Could you check a few things on this model? Use its own coordinates, in mm. A direction names the side the tool comes from. Round coordinates to 2 decimals unless told otherwise and drop trailing zeros. Write each loop counter-clockwise with the first axis right and the second up, starting at its lowest first coordinate (ties: lowest second). Pieces come first, ordered by that corner, then holes. Notation, with made-up numbers: (32.25, -36) - (66.25, -36) arc R24 cw to (66.25, -12) - close; hole circle Ø1 at (61, 29). An arc over 180 degrees is marked (long way). Put each result on its own line as item: value.
from build123d import *

# Parameters (mm, degrees)
F0_W     = 27
F0_H     = 27
F0_R     = 1.75
F1_DEPTH = 3
F2_R     = 8.5
F3_DEPTH = 3


with BuildPart() as f1:
    # F0 (on Front) → F1 (new body)
    with BuildSketch(Plane.XZ):
        Rectangle(F0_W, F0_H)
        with Locations((-10.5, -10.5)):
            Circle(F0_R, mode=Mode.SUBTRACT)
        with Locations((10.5, -10.5)):
            Circle(F0_R, mode=Mode.SUBTRACT)
        with Locations((-10.5, 10.5)):
            Circle(F0_R, mode=Mode.SUBTRACT)
        with Locations((10.5, 10.5)):
            Circle(F0_R, mode=Mode.SUBTRACT)
    extrude(amount=F1_DEPTH)

    # F2 (on face) → F3 (join)
    with BuildSketch(Plane.XZ.offset(3)):
        Circle(F2_R)
    extrude(amount=F3_DEPTH)


solid = f1.part
(1) Imagine slicing it at C-C, the plane z = 10.5. List the corners of the cut face in (x, y) for me.
Values found:
outline: (-13.5, -3) - (-12.25, -3) - (-12.25, 0) - (-13.5, 0) - close; (-8.75, -3) - (8.75, -3) - (8.75, 0) - (-8.75, 0) - close; (12.25, -3) - (13.5, -3) - (13.5, 0) - (12.25, 0) - close
(2) For faces 4 (the face through (-6.2, -3, 6.2)), 5 (the face through (-10.728, -1.479, -8.765)), which set-ups out of +Z, -Z, +X, -X, +Y, -Y let a thin tool reach every point of the face, with its end or its side?
Values found:
face 4: -Y
face 5: +Y, -Y
(3) I'm going to push flat-ended pins straight in: pin 1 (1.5 mm diameter, centred on x = 7.5, y = -4, fed in from +Z); pin 2 (1.5 mm diameter, centred on x = 1, y = -4.5, fed in from +Z); pin 3 (4 mm diameter, centred on x = 10.5, z = -10.5, fed in from +Y); pin 4 (1 mm diameter, centred on x = -3.5, y = -4.5, fed in from -Z). Where does each tip first touch, or does it pass through?
Values found:
pin 1: stops at z = 5.17
pin 2: stops at z = 8.5
pin 3: stops at y = 0
pin 4: stops at z = -7.95
(4) Imagine slicing it at A-A, the plane x = -10.5. List the corners of the cut face in (y, z) for me.
Values found:
outline: (-3, -13.5) - (0, -13.5) - (0, -12.25) - (-3, -12.25) - close; (-3, -8.75) - (0, -8.75) - (0, 8.75) - (-3, 8.75) - close; (-3, 12.25) - (0, 12.25) - (0, 13.5) - (-3, 13.5) - close
(5) If we mould it in two halves opening along Z, with no side actions, what happens to faces 1 (the face through (0, -1, -13.5)), 2 (the face through (0, -6, 0)), 3 (the face through (11.4, -1.5, 12))? For each: pulls with the +Z half, pulls with the -Z half, needs draft (parallel to the pull), parting line crosses it, or undercut.
Values found:
face 1: pulls with the -Z half
face 2: needs draft
face 3: undercut
(6) Please list where these lines run through material, in increasing order: probe 1 along Z at (x, y) = (10.5, -1.2); probe 2 along X at (y, z) = (-1.9, -10); probe 3 along Z at (x, y) = (9.5, -0.4). Write a range as from..to.
Values found:
probe 1: z = -13.5..-12.25, -8.75..8.75, 12.25..13.5
probe 2: x = -13.5..-12.18, -8.82..8.82, 12.18..13.5
probe 3: z = -13.5..-11.94, -9.06..9.06, 11.94..13.5
(7) Imagine slicing it at D-D, the plane z = 0. List the corners of the cut face in (x, y) for me, then the cut area to 3 significant figures.
Values found:
outline: (-13.5, -3) - (-8.5, -3) - (-8.5, -6) - (8.5, -6) - (8.5, -3) - (13.5, -3) - (13.5, 0) - (-13.5, 0) - close
area: 132 mm^2
(8) Imagine slicing it at B-B, the plane y = -0.95. List the corners of the cut face in (x, z) for me, then the cut area to 3 significant figures.
Values found:
outline: (-13.5, -13.5) - (13.5, -13.5) - (13.5, 13.5) - (-13.5, 13.5) - close; hole circle Ø3.5 at (-10.5, -10.5); hole circle Ø3.5 at (-10.5, 10.5); hole circle Ø3.5 at (10.5, -10.5); hole circle Ø3.5 at (10.5, 10.5)
area: 691 mm^2
